from build123d import *

# Parameters (mm, degrees)
CROQUIS1_R              = 31
SALIENTE_EXTRUIR1_DEPTH = 2
CROQUIS2_R              = 28
SALIENTE_EXTRUIR2_DEPTH = 10
CROQUIS3_R              = 11.5
CORTAR_EXTRUIR1_DEPTH   = 20
CROQUIS4_R              = 17.5
CORTAR_EXTRUIR2_DEPTH   = 3


with BuildPart() as part:
    # Croquis1 → Saliente-Extruir1 (new body)
    with BuildSketch(Plane.XY):
        Circle(CROQUIS1_R)
    extrude(amount=SALIENTE_EXTRUIR1_DEPTH)

    # Croquis2 → Saliente-Extruir2 (add)
    with BuildSketch(Plane.XY.offset(2)):
        Circle(CROQUIS2_R)
    extrude(amount=SALIENTE_EXTRUIR2_DEPTH)

    # Croquis3 → Cortar-Extruir1 (cut)
    with BuildSketch(Plane.XY.offset(12)):
        Circle(CROQUIS3_R)
    extrude(amount=-CORTAR_EXTRUIR1_DEPTH, mode=Mode.SUBTRACT)

    # Croquis4 → Cortar-Extruir2 (cut)
    with BuildSketch(Plane.XY.offset(12)):
        Circle(CROQUIS4_R)
    extrude(amount=-CORTAR_EXTRUIR2_DEPTH, mode=Mode.SUBTRACT)


solid = part.part
The model under review builds one solid part; all positions refer to its coordinate system, in mm. A direction names the side the tool comes from. Coordinates: 2 decimals unless noted, no trailing zeros. Order: outer loops, then holes, each group sorted by start corner. A loop starts at its lowest first (then second) coordinate and runs counter-clockwise, first axis right, second up. Notation, with made-up numbers: (12.25, 63) -> (48.25, 63) arc R30 cw to (48.25, 102) -> close; hole circle Ø1 at (-12, 36). An arc over 180 degrees is marked (long way). Answer in a Markdown table with one row per item.
(1) Consider section A-A (x = 0). Write out the cut boundary in (y, z).
Answers:
| item | result |
|---|---|
| outline | (-31, 0) -> (-11.5, 0) -> (-11.5, 9) -> (-17.5, 9) -> (-17.5, 12) -> (-28, 12) -> (-28, 2) -> (-31, 2) -> close; (11.5, 0) -> (31, 0) -> (31, 2) -> (28, 2) -> (28, 12) -> (17.5, 12) -> (17.5, 9) -> (11.5, 9) -> close |
(2) Machinability: for faces 1 (the cylindrical face through (-4.036, 30.736, 0.986)), 2 (the flat face through (-7, -27.4, 2)), which of the approach directions +Z, -Z, +X, -X, +Y, -Y give a long, thin tool a straight path to every point of the face, cutting with its end or side? Answer none if there is none.
Answers:
| item | result |
|---|---|
| face 1 | +Z, -Z |
| face 2 | +Z |
(3) Consider section C-C (z = 6). Write out the cut boundary in (x, y), plus the area to 3 significant figures.
Answers:
| item | result |
|---|---|
| outline | circle Ø56 at (0, 0); hole circle Ø23 at (0, 0) |
| area | 2,050 mm² |
(4) Insertion check: pin 1 (1.5 mm diameter, centred on x = -15, z = 8, fed in from -Y); pin 2 (17.5 mm diameter, centred on x = 1.5, y = 8.5, fed in from +Z); pin 3 (18.5 mm diameter, centred on x = 0, y = 0, fed in from +Z); pin 4 (3 mm diameter, centred on y = 23, z = 6, fed in from +X). Each pin has a flat end and moves straight along its axis. Give the tip position at first contact, or say it passes through.
Answers:
| item | result |
|---|---|
| pin 1 | y = -24.1 |
| pin 2 | z = 9 |
| pin 3 | through |
| pin 4 | x = 17.94 |
(5) The part is to be moulded in two halves that separate along Y. For faces 3 (the cylindrical face through (-1.5, 11.4, 4.6)), 4 (the cylindrical face through (25.865, -10.724, 6.93)), 5 (the flat face through (-13, -12, 12)), 6 (the flat face through (4, -11, 9)), say which applies: +Y half, -Y half, draft (parallel to the pull), parting line (faces both ways), or undercut.
Answers:
| item | result |
|---|---|
| face 3 | undercut |
| face 4 | parting line |
| face 5 | draft |
| face 6 | undercut |
(6) Wall thickness on line 1 along Y through (x, z) = (0, 3.5); line 2 along X through (y, z) = (0.5, 0.5); line 3 along Y through (x, z) = (0, 10.4): over which ranges is each line inside the solid? List them lowest first.
Answers:
| item | result |
|---|---|
| line 1 | -28 to -11.5, 11.5 to 28 |
| line 2 | -31 to -11.49, 11.49 to 31 |
| line 3 | -28 to -17.5, 17.5 to 28 |
(7) Consider section D-D (y = -27). Write out the cut boundary in (x, z).
Answers:
| item | result |
|---|---|
| outline | (-15.23, 0) -> (15.23, 0) -> (15.23, 2) -> (7.42, 2) -> (7.42, 12) -> (-7.42, 12) -> (-7.42, 2) -> (-15.23, 2) -> close |
